The listing builds one solid part. Answer for the finished solid, in the listing's coordinates (mm). Face numbers are marked on the shaded views. A direction names the side the tool comes from. Round coordinates to 2 decimals unless told otherwise and drop trailing zeros. Write each loop counter-clockwise with the first axis right and the second up, starting at its lowest first coordinate (ties: lowest second). Pieces come first, ordered by that corner, then holes. Notation, with made-up numbers: M -30,56.5 L 5,56.5 A8 cw 5,68.5 Z; hole C 51,-16 d5. An arc over 180 degrees is marked long. Write each question's results on one line, items separated by ' | '.
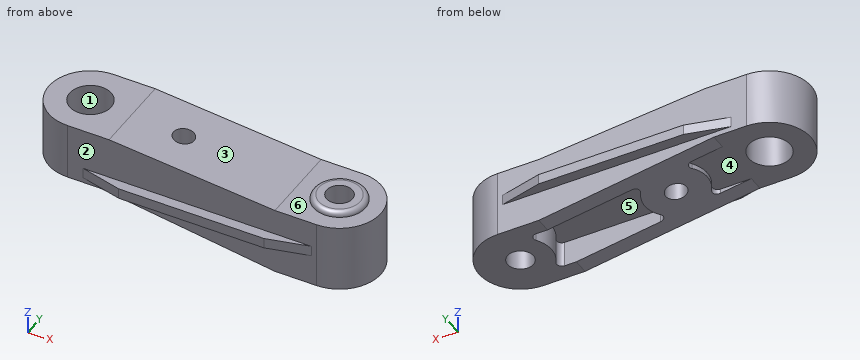
from build123d import *

# Parameters (mm, degrees)
BASE_EXTRUSION_DEPTH    = 4.5
BOSS_EXTRU_1_DEPTH      = 0.5
ENL_V_MAT_EXTRU_1_DEPTH = 30.753151094
ENL_V_MAT_EXTRU_2_DEPTH = 30.753151094
ESQUISSE5_R             = 1.25
ESQUISSE5_R_2           = 1
ENL_V_MAT_EXTRU_3_DEPTH = 30.546573405
ESQUISSE11_R            = 2.5
BOSS_EXTRU_2_DEPTH      = 0.5
CONG_1_R                = 0.5
ESQUISSE12_R            = 1.25
ENL_V_MAT_EXTRU_5_DEPTH = 30.291637032
ESQUISSE13_R            = 2
ENL_V_MAT_EXTRU_6_DEPTH = 30.546573405
ENL_V_MAT_EXTRU_7_DEPTH = 2.5


with BuildPart() as part:
    # Esquisse1 → Base-Extrusion (new, symmetric)
    with BuildSketch(Plane.XY):
        with BuildLine():
            Line((0, 4), (24, 4))
            ThreePointArc((24, 4), (28, 0), (24, -4))
            Line((24, -4), (0, -4))
            ThreePointArc((0, -4), (-4, 0), (0, 4))
        make_face()
    extrude(amount=BASE_EXTRUSION_DEPTH, both=True)

    # Esquisse2 → Boss.-Extru.1 (add, symmetric)
    with BuildSketch(Plane.XY):
        Polygon((5.5, 5), (1.5, 4), (1.5, -4), (5.5, -5), (19.5, -5), (23.5, -4), (23.5, 4), (19.5, 5), align=None)
    extrude(amount=BOSS_EXTRU_1_DEPTH, both=True)

    # Esquisse3 → Enlèv. mat.-Extru.1 (cut, through all)
    with BuildSketch(Plane.XZ.offset(4)):
        Polygon((29, 3), (20, 3), (4.013550136, 4.5), (-6, 4.5), (-6, 6), (29, 6), align=None)
    extrude(amount=-ENL_V_MAT_EXTRU_1_DEPTH, mode=Mode.SUBTRACT)

    # Esquisse4 → Enlèv. mat.-Extru.2 (cut, through all)
    with BuildSketch(Plane.XZ.offset(4)):
        Polygon((-6, -1), (3.145079466, -1), (20, -3.5), (29.207616232, -3.5), (29.207616232, -4.5), (29.207616232, -7.5), (-6, -7.5), align=None)
    extrude(amount=-ENL_V_MAT_EXTRU_2_DEPTH, mode=Mode.SUBTRACT)

    # Esquisse5 → Enlèv. mat.-Extru.3 (cut, through all)
    with BuildSketch(Plane.XY.offset(4.5)):
        with Locations((24, 0)):
            Circle(ESQUISSE5_R)
        with Locations(Location((9, 0, 0), (0, 0, 180))):
            Circle(ESQUISSE5_R_2)
    extrude(amount=-ENL_V_MAT_EXTRU_3_DEPTH, mode=Mode.SUBTRACT)

    # Esquisse11 → Boss.-Extru.2 (add)
    with BuildSketch(Plane.XY.offset(3)):
        with Locations((24, 0)):
            Circle(ESQUISSE11_R)
    extrude(amount=BOSS_EXTRU_2_DEPTH)

    # Congé1
    cong_1_edges = [part.edges().sort_by_distance(p)[0] for p in [
        (21.5, 0, 3.5),
    ]]
    fillet(cong_1_edges, radius=CONG_1_R - 0.0001)  # a hair under: the kernel refuses the full size

    # Esquisse12 → Enlèv. mat.-Extru.5 (cut, through all)
    with BuildSketch(Plane.XY.offset(3.5)):
        with Locations((24, 0)):
            Circle(ESQUISSE12_R)
    extrude(amount=-ENL_V_MAT_EXTRU_5_DEPTH, mode=Mode.SUBTRACT)

    # Esquisse13 → Enlèv. mat.-Extru.6 (cut, through all)
    with BuildSketch(Plane.XY.offset(4.5)):
        Circle(ESQUISSE13_R)
    extrude(amount=-ENL_V_MAT_EXTRU_6_DEPTH, mode=Mode.SUBTRACT)

    # Esquisse14 → Enlèv. mat.-Extru.7 (cut)
    with BuildSketch(Plane(origin=(0, 0, -3.5), x_dir=(-1, 0, 0), z_dir=(0, 0, -1))):
        with BuildLine():
            Line((-2.872281323, 2.5), (-6.127718677, 2.5))
            ThreePointArc((-6.127718677, 2.5), (-6.570921307, 2.231455025), (-6.53804458, 1.714285714))
            ThreePointArc((-6.53804458, 1.714285714), (-6, 0), (-6.53804458, -1.714285714))
            ThreePointArc((-6.53804458, -1.714285714), (-6.570921307, -2.231455025), (-6.127718677, -2.5))
            Line((-6.127718677, -2.5), (-2.872281323, -2.5))
            ThreePointArc((-2.872281323, -2.5), (-2.429078693, -2.231455025), (-2.46195542, -1.714285714))
            ThreePointArc((-2.46195542, -1.714285714), (-3, 0), (-2.46195542, 1.714285714))
            ThreePointArc((-2.46195542, 1.714285714), (-2.429078693, 2.231455025), (-2.872281323, 2.5))
        make_face()
        with BuildLine():
            Line((-11.872281323, -2.5), (-21.127718677, -2.5))
            ThreePointArc((-21.127718677, -2.5), (-21.570921307, -2.231455025), (-21.53804458, -1.714285714))
            ThreePointArc((-21.53804458, -1.714285714), (-21, 0), (-21.53804458, 1.714285714))
            ThreePointArc((-21.53804458, 1.714285714), (-21.570921307, 2.231455025), (-21.127718677, 2.5))
            Line((-21.127718677, 2.5), (-11.872281323, 2.5))
            ThreePointArc((-11.872281323, 2.5), (-11.429078693, 2.231455025), (-11.46195542, 1.714285714))
            ThreePointArc((-11.46195542, 1.714285714), (-12, 0), (-11.46195542, -1.714285714))
            ThreePointArc((-11.46195542, -1.714285714), (-11.429078693, -2.231455025), (-11.872281323, -2.5))
        make_face()
    extrude(amount=-ENL_V_MAT_EXTRU_7_DEPTH, mode=Mode.SUBTRACT)


solid = part.part
1) Section B-B (y = 0) is taken. State how many separate pieces and enclosed holes the cut face has, then the cut area to 3 significant figures.
Return value:
separate pieces: 4 | enclosed holes: 0 | area: 126 mm²
2) Section D-D (z = -2.75) is taken. Determine the outline of the cut face in (x, y), then the cut area to 3 significant figures.
Return value:
outline: M 14.94,-4 L 24,-4 A4 ccw 24,4 L 14.94,4 L 14.94,2.5 L 21.13,2.5 A0.5 cw 21.54,1.71 A3 ccw 21.54,-1.71 A0.5 cw 21.13,-2.5 L 14.94,-2.5 Z; hole C 24,0 d2.5 | area: 60.9 mm²
3) Find the intervals of material crossed by line 1 (Y direction, x = 24, z = 0.75); line 2 (Y direction, x = 9, z = 1.25); line 3 (Y direction, x = 19, z = 2.5), in increasing order.
Return value:
line 1: -4 to -1.25, 1.25 to 4 | line 2: -4 to -1, 1 to 4 | line 3: -4 to 4
4) Section A-A (z = 1) is taken. Determine the outline of the cut face in (x, y).
Return value:
outline: M 0,-4 L 24,-4 A4 ccw 24,4 L 0,4 A4 ccw Z; hole C 0,0 d4; hole C 9,0 d2; hole C 24,0 d2.5
5) Each of these flat-tipped pins is pushed along its axis until it touches: pin 1 (2.5 mm diameter, centred on x = 18, z = 2, fed in from -Y); pin 2 (1.1 mm diameter, centred on x = 12, y = 4.5, fed in from +Z); pin 3 (1 mm diameter, centred on x = 5.5, y = -4, fed in from +Z); pin 4 (3 mm diameter, centred on x = 24, y = 0, fed in from -Z). Where does it stop, or does it pass through?
Return value:
pin 1: y = -4 | pin 2: z = 3.77 | pin 3: z = 4.41 | pin 4: z = -3.5
6) A tool of negligible diameter and unlimited length cuts with its end or side. For the marked faces 4, 5 and 6, from which of +Z, -Z, +X, -X, +Y, -Y can it reach the whole face along a straight path? Write none if from no direction.
Return value:
face 4: -Z, -X | face 5: -Z | face 6: +Z
7) The mould has two halves that part along Y. Classify the marked faces 1, 2 and 3: +Y half, -Y half, draft (parallel to the pull), parting line (faces both ways), or undercut.
Return value:
face 1: undercut | face 2: -Y half | face 3: draft
8) Section C-C (x = 9) is taken. Determine the outline of the cut face in (y, z), then the cut area to 3 significant figures.
Return value:
outline: M -5,-0.5 L -4,-0.5 L -4,-1.87 L -1,-1.87 L -1,4.03 L -4,4.03 L -4,0.5 L -5,0.5 Z; M 1,-1.87 L 4,-1.87 L 4,-0.5 L 5,-0.5 L 5,0.5 L 4,0.5 L 4,4.03 L 1,4.03 Z | area: 37.4 mm²
